```python
from build123d import *

# Parameters (mm, degrees)
F0_R     = 3.048
F1_DEPTH = 4.7625
F2_R     = 4.7625
F3_DEPTH = 9.525
F5_DEPTH = 0.79375
F6_R     = 0.396875


with BuildPart() as f1:
    # F0 (on Top) → F1 (new body, symmetric)
    with BuildSketch(Plane.XY):
        Circle(F0_R)
    extrude(amount=F1_DEPTH, both=True)

    # F2 (on face) → F3 (join)
    with BuildSketch(Plane.XY.offset(4.7625)):
        Circle(F2_R)
    extrude(amount=F3_DEPTH)

    # F4 (on face) → F5 (cut)
    with BuildSketch(Plane.XY.offset(14.2875)):
        with BuildLine():
            ThreePointArc((0.9652, 3.0247337007), (0.0066610182, 3.1749930127), (-0.9525, 3.0287569645))
            Line((-0.9525, 3.0287569645), (-0.9525, 0.9652))
            Line((-0.9525, 0.9652), (-3.0247337007, 0.9652))
            ThreePointArc((-3.0247337007, 0.9652), (-3.1749930127, 0.0066610182), (-3.0287569645, -0.9525))
            Line((-3.0287569645, -0.9525), (-0.9525, -0.9525))
            Line((-0.9525, -0.9525), (-0.9525, -3.0287569645))
            ThreePointArc((-0.9525, -3.0287569645), (0.0066610182, -3.1749930127), (0.9652, -3.0247337007))
            Line((0.9652, -3.0247337007), (0.9652, -0.9525))
            Line((0.9652, -0.9525), (3.0287569645, -0.9525))
            ThreePointArc((3.0287569645, -0.9525), (3.1749930127, 0.0066610182), (3.0247337007, 0.9652))
            Line((3.0247337007, 0.9652), (0.9652, 0.9652))
            Line((0.9652, 0.9652), (0.9652, 3.0247337007))
        make_face()
    extrude(amount=-F5_DEPTH, mode=Mode.SUBTRACT)

    # F6
    f6_edges = [f1.edges().sort_by_distance(p)[0] for p in [
        (-0.9525, 0.9652, 13.890625),
        (0.9652, 0.9652, 13.890625),
        (0.9652, -0.9525, 13.890625),
        (-0.9525, -0.9525, 13.890625),
        (-3.028757, -0.9525, 13.890625),
        (-3.024734, 0.9652, 13.890625),
        (0.9652, -3.024734, 13.890625),
        (3.028757, -0.9525, 13.890625),
        (3.024734, 0.9652, 13.890625),
        (0.9652, 3.024734, 13.890625),
        (-0.9525, 3.028757, 13.890625),
        (-0.9525, -3.028757, 13.890625),
    ]]
    fillet(f6_edges, radius=F6_R)


solid = f1.part
```
CAD build for the part. Positions are in the model's coordinates, mm. Round coordinates to 2 decimals unless told otherwise and drop trailing zeros. Order: outer loops, then holes, each group sorted by start corner. A loop starts at its lowest first (then second) coordinate and runs counter-clockwise, first axis right, second up.
Item 1: Mould opens along Y. For faces 1 (the face through (0, 0, 13.494)), 2 (the face through (1, -3.1, 4.762)), 3 (the face through (-0.4, 3.02, 0.07)) say: pulls with the +Y half, pulls with the -Y half, needs draft (parallel to the pull), parting line crosses it, or undercut.
Item 2: Saw through at D-D on z = 2.5. Write the cut outline in (x, y), then the cut area to 3 significant figures.
Item 3: Probe line 1 along Z through (x, y) = (3, -2.5); line 2 along Z through (x, y) = (-1.5, 0.5); line 3 along X through (y, z) = (-2.75, -0.25). List the from-to ranges inside material, lowest first.
Item 4: Pin check, flat tips, straight feed: pin 1 (3 mm diameter, centred on y = -2, z = 6.5, fed in from +X); pin 2 (0.6 mm diameter, centred on y = -2, z = 14, fed in from +X); pin 3 (0.9 mm diameter, centred on x = -2, z = 14, fed in from -Y). Stop position of each tip, or through.
Item 5: Saw through at C-C on z = 5. Write the cut outline in (x, y) (1 decimal).
Item 6: Saw through at A-A on y = 0. Write the cut outline in (x, z) (1 decimal), then the cut area to 3 significant figures.
Reported:
1. face 1: undercut
1. face 2: needs draft
1. face 3: parting line crosses it
2. outline: circle Ø6.1 at (0, 0)
2. area: 29.2 mm2
3. line 1: z = 4.76 to 14.29
3. line 2: z = -4.76 to 13.49
3. line 3: x = -1.31 to 1.31
4. pin 1: stops at x = 4.74
4. pin 2: stops at x = 4.45
4. pin 3: stops at y = -4.5
5. outline: circle Ø9.5 at (0, 0)
6. outline: (-4.8, 4.8) - (-3, 4.8) - (-3, -4.8) - (3, -4.8) - (3, 4.8) - (4.8, 4.8) - (4.8, 14.3) - (3.2, 14.3) - (3.2, 13.5) - (-3.2, 13.5) - (-3.2, 14.3) - (-4.8, 14.3) - close
6. area: 144 mm2
